from build123d import *

# Parameters (mm, degrees)
SKETCH1_W           = 325
SKETCH1_H           = 260
BOSS_EXTRUDE1_DEPTH = 80
SKETCH2_R           = 65
CUT_EXTRUDE1_DEPTH  = 61.2
SKETCH3_R           = 42
CUT_EXTRUDE2_DEPTH  = 424.821896556
SKETCH4_W           = 325
SKETCH4_H           = 260
SKETCH4_W_2         = 247
SKETCH4_H_2         = 232
CUT_EXTRUDE3_DEPTH  = 66


with BuildPart() as part:
    # Sketch1 → Boss-Extrude1 (new body)
    with BuildSketch(Plane.XY):
        with Locations((162.5, 130)):
            Rectangle(SKETCH1_W, SKETCH1_H)
    extrude(amount=-BOSS_EXTRUDE1_DEPTH)

    # Sketch2 → Cut-Extrude1 (cut)
    with BuildSketch(Plane.XY):
        with Locations((162.5, 130)):
            Circle(SKETCH2_R)
    extrude(amount=-CUT_EXTRUDE1_DEPTH, mode=Mode.SUBTRACT)

    # Sketch3 → Cut-Extrude2 (cut, through all)
    with BuildSketch(Plane.XY):
        with Locations((162.5, 130)):
            Circle(SKETCH3_R)
    extrude(amount=-CUT_EXTRUDE2_DEPTH, mode=Mode.SUBTRACT)

    # Sketch4 → Cut-Extrude3 (cut)
    with BuildSketch(Plane(origin=(0, 0, -80), x_dir=(-1, 0, 0), z_dir=(0, 0, -1))):
        with Locations((-162.5, 130)):
            Rectangle(SKETCH4_W, SKETCH4_H)
        with Locations((-162.5, 130)):
            Rectangle(SKETCH4_W_2, SKETCH4_H_2, mode=Mode.SUBTRACT)
    extrude(amount=-CUT_EXTRUDE3_DEPTH, mode=Mode.SUBTRACT)


solid = part.part
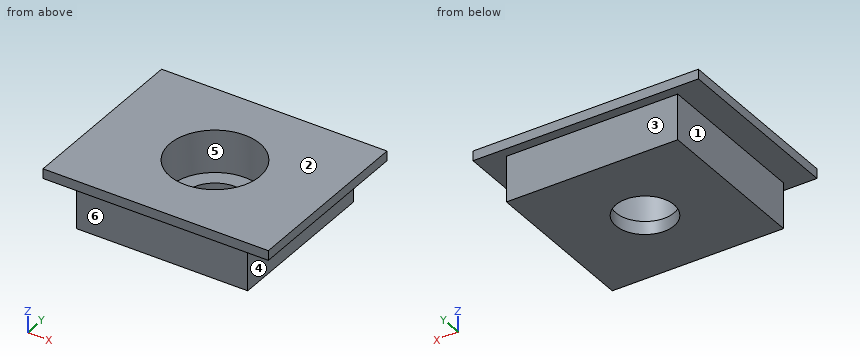
For this review, take the finished solid that the model builds, in its own axes (mm). Face numbers are marked on the shaded views. A direction names the side the tool comes from. Round coordinates to 2 decimals unless told otherwise and drop trailing zeros. Write each loop counter-clockwise with the first axis right and the second up, starting at its lowest first coordinate (ties: lowest second). Pieces come first, ordered by that corner, then holes. Notation, with made-up numbers: (28, 29.5) - (86, 29.5) arc R31 cw to (86, 56.5) - close; hole circle Ø7 at (-39, 43). An arc over 180 degrees is marked (long way). Write item = value, one per line. Start each with the question number.
1. Consider section B-B on y = 130. State the section outline as (x, z) points, plus the area to 3 significant figures.
2. Consider section D-D on y = 23. State the section outline as (x, z) points, plus the area to 3 significant figures.
3. Consider section A-A on x = 162.5. State the section outline as (y, z) points.
4. For pin 1 Ø10 at (y, z) = (168, -40) entering from -X; pin 2 Ø6 at (y, z) = (233.5, -64.5) entering from +X; pin 3 Ø2 at (x, z) = (257, -43.5) entering from +Y, all flat-tipped, find the tip position at first contact; note any pin that passes through.
5. Wall thickness on L1, parallel to Y at x = 162, z = -31; L2, parallel to Y at x = 162, z = -65; L3, parallel to Z at x = 117.5, y = 127: over which ranges is each line inside the solid? List them lowest first.
6. Draft analysis for pull direction X (two halves, no side actions). For the marked faces 4, 5 and 6, state which applies: released by +X, released by -X, zero draft, split by the parting line, or undercut.
7. Consider section C-C on z = -52.5. State the section outline as (x, y) points, plus the area to 3 significant figures.
8. For the marked faces 1, 2 and 3, list the 3-axis set-ups (+Z, -Z, +X, -X, +Y, -Y) from which the entire face can be reached by the end or side of a thin tool; tool diameter is ignored.
Evaluation:
q1.outline = (0, -14) - (39, -14) - (39, -80) - (120.5, -80) - (120.5, -61.2) - (97.5, -61.2) - (97.5, 0) - (0, 0) - close; (204.5, -80) - (286, -80) - (286, -14) - (325, -14) - (325, 0) - (227.5, 0) - (227.5, -61.2) - (204.5, -61.2) - close
q1.area = 11,300 mm2
q2.outline = (0, -14) - (39, -14) - (39, -80) - (286, -80) - (286, -14) - (325, -14) - (325, 0) - (0, 0) - close
q2.area = 20,900 mm2
q3.outline = (0, -14) - (14, -14) - (14, -80) - (88, -80) - (88, -61.2) - (65, -61.2) - (65, 0) - (0, 0) - close; (172, -80) - (246, -80) - (246, -14) - (260, -14) - (260, 0) - (195, 0) - (195, -61.2) - (172, -61.2) - close
q4.pin_1 = 39
q4.pin_2 = 286
q4.pin_3 = 246
q5.L1 = 14 to 65, 195 to 246
q5.L2 = 14 to 88, 172 to 246
q5.L3 = -80 to -61.2
q6.face_4 = released by +X
q6.face_5 = undercut
q6.face_6 = zero draft
q7.outline = (39, 14) - (286, 14) - (286, 246) - (39, 246) - close; hole circle Ø130 at (162.5, 130)
q7.area = 44,000 mm2
q8.face_1 = -Z, -X, +Y, -Y
q8.face_2 = +Z, +X, -X, +Y, -Y
q8.face_3 = -Z, +X, -X, +Y
